Input: dimensioned drawing with shaded views. Units: mm. Origin: part minimum x, y, z. A direction names the side the tool comes from. Give positions to 0.01 mm unless a question says otherwise; leave off trailing zeros. Order: outer loops, then holes, each group sorted by start corner. A loop starts at its lowest first (then second) coordinate and runs counter-clockwise, first axis right, second up.
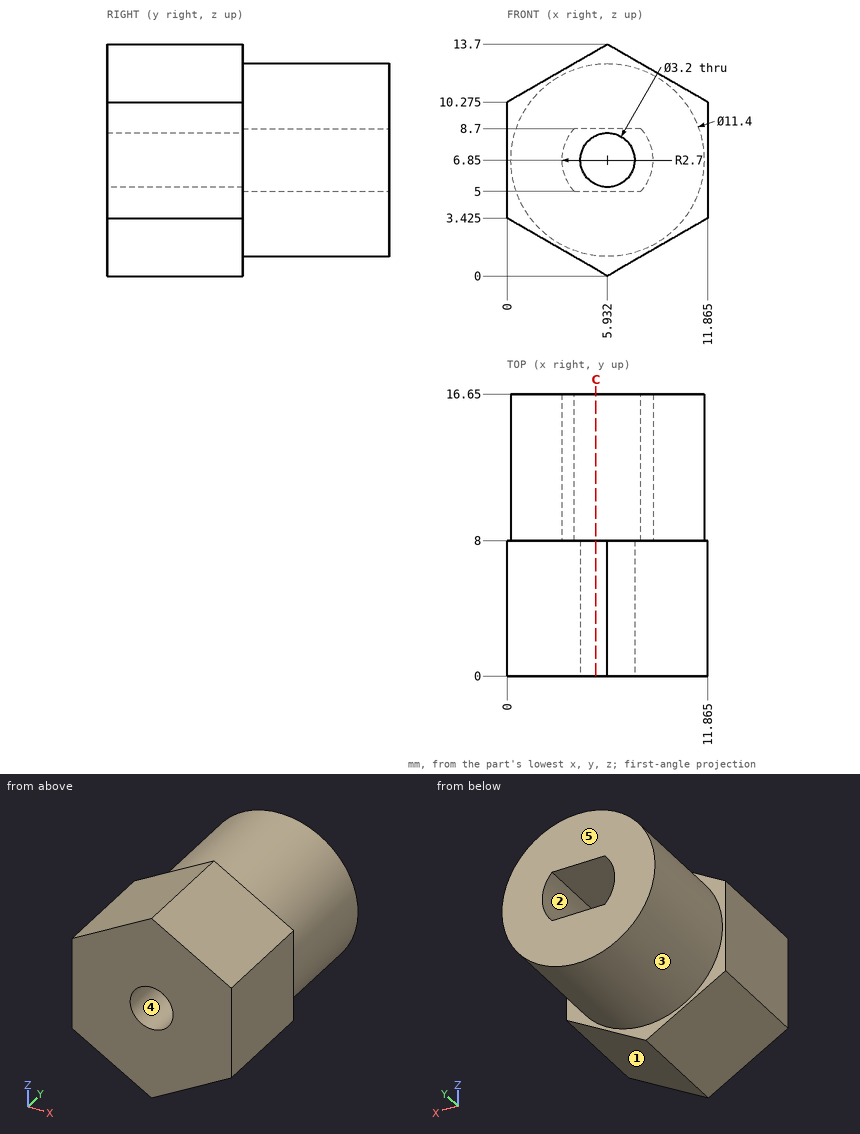
1) Pin query (flat end, axial travel): pin 1 (8 mm diameter, centred on y = 12.5, z = 10.5, fed in from -X); pin 2 (1.5 mm diameter, centred on x = 1.5, y = 10, fed in from -Z); pin 3 (3 mm diameter, centred on x = 6.5, y = 10.5, fed in from +Z). Return the tip coordinate at first contact, or that it passes through.
Report:
pin 1: stops at x = 0.23
pin 2: stops at z = 2.5
pin 3: stops at z = 12.55
2) Draft query along Z for the marked faces 3, 4 and 5. Return one class per face: +Z half, -Z half, draft (parallel to the pull), parting line (faces both ways), or undercut.
Report:
face 3: parting line
face 4: undercut
face 5: draft
3) Reachability of the marked faces 1 and 2 from +Z, -Z, +X, -X, +Y, -Y: full face, straight path, thin tool, end or side. Return the list, or none.
Report:
face 1: -Z, +X, +Y, -Y
face 2: +Y
4) Section query C-C, the plane x = 5.25. Return the cut outline in (y, z).
Report:
outline: (0, 0.39) - (8, 0.39) - (8, 1.19) - (16.65, 1.19) - (16.65, 5) - (8, 5) - (8, 5.4) - (0, 5.4) - close; (0, 8.3) - (8, 8.3) - (8, 8.7) - (16.65, 8.7) - (16.65, 12.51) - (8, 12.51) - (8, 13.31) - (0, 13.31) - close
5) Material intervals for L1, parallel to X at y = 2, z = 6.85 (1 decimal); L2, parallel to Y at x = 6, z = 13; L3, parallel to X at y = 9, z = 7.5 (1 decimal), sorted ascending.
Report:
L1: x = 0 to 4.3, 7.5 to 11.9
L2: y = 0 to 8
L3: x = 0.3 to 3.3, 8.6 to 11.6
